Check sheet for the modelled part. Datum: model origin and axes. Units: mm. Face numbers are marked on the shaded views. A direction names the side the tool comes from. Round coordinates to 2 decimals unless told otherwise and drop trailing zeros. Write each loop counter-clockwise with the first axis right and the second up, starting at its lowest first coordinate (ties: lowest second). Pieces come first, ordered by that corner, then holes. Notation, with made-up numbers: (84, 12.5) -> (141, 12.5) arc R29 cw to (141, 36.5) -> close; hole circle Ø9 at (-19.75, 87). An arc over 180 degrees is marked (long way). Write item = value, one per line.
from build123d import *

# Parameters (mm, degrees)
F0_W           = 21
F0_H           = 36.8
F0_R           = 2
F1_DEPTH       = 0.8
F0_W_2         = 5
F2_DEPTH       = 13.5
F5_R           = 6.35
F6_D           = 5
F6_CBORE_D     = 9.5
F6_CBORE_DEPTH = 4.2
F7_W           = 10.5
F7_H           = 2
F7_R           = 2
F8_DEPTH       = 2
F9_DEPTH       = 6.35
F10_T4_DEPTH   = 35.8364431643
F10_T9_DEPTH   = 35.8364431643
F11_W          = 6.8
F11_H          = 6.8
F12_DEPTH      = 2
F13_R          = 0.99999


# Not quite as in the source:
# - a fillet or chamfer that OpenCascade refuses, or shapes differently, is made with other operations: its cross-section is extruded or revolved along the edge and cut away or added
# - a fillet or chamfer is up to 0.001 mm smaller than in the source, because OpenCascade refuses the exact size


with BuildPart() as f1:
    # F0 (on Top) → F1 (new body)
    with BuildSketch(Plane.XY):
        Rectangle(F0_W, F0_H)
        with Locations((-6.35, -12.7)):
            Circle(F0_R, mode=Mode.SUBTRACT)
        with Locations((6.35, -12.7)):
            Circle(F0_R, mode=Mode.SUBTRACT)
        with Locations((-6.35, 12.7)):
            Circle(F0_R, mode=Mode.SUBTRACT)
        with Locations((6.35, 12.7)):
            Circle(F0_R, mode=Mode.SUBTRACT)
    extrude(amount=F1_DEPTH)

    # F0 (on Top) → F2 (join)
    with BuildSketch(Plane.XY):
        with Locations((-13, 0)):
            Rectangle(F0_W_2, F0_H)
    extrude(amount=F2_DEPTH)

    # F5
    f5_edges = [f1.edges().sort_by_distance(p)[0] for p in [
        (-13, -18.4, 13.5),
        (-13, 18.4, 13.5),
    ]]
    fillet(f5_edges, radius=F5_R)

    # F6 (through all)
    with Locations(Plane.YZ.offset(-10.5)):
        with Locations((0, 7.15)):
            CounterBoreHole(F6_D / 2, F6_CBORE_D / 2, F6_CBORE_DEPTH)

    # F7 (on face) → F8 (join)
    with BuildSketch(Plane.XY.offset(0.8)):
        with Locations((-5.25, -17.4)):
            Rectangle(F7_W, F7_H)
        Polygon((-10.5, -16.4), (0, -16.4), (0, -18.4), (10.5, -18.4), (10.5, -7), (-10.5, -7), align=None)
        Polygon((-10.5, 16.4), (-10.5, 7), (10.5, 7), (10.5, 18.4), (0, 18.4), (0, 16.4), align=None)
        with Locations((-6.35, 12.7)):
            Circle(F7_R, mode=Mode.SUBTRACT)
        with Locations((6.35, 12.7)):
            Circle(F7_R, mode=Mode.SUBTRACT)
    extrude(amount=F8_DEPTH)

    # F7 (on face) → F9 (join)
    with BuildSketch(Plane.XY.offset(0.8)):
        with Locations((-5.25, -17.4)):
            Rectangle(F7_W, F7_H)
        with Locations((-5.25, 17.4)):
            Rectangle(F7_W, F7_H)
    extrude(amount=F9_DEPTH)

    # F10: chamfer of 6.35 x 6.5756174926 on 2 edges, made by hand


with BuildPart() as f10_tool2:
    # F10_s3 → F10_t4 (new body)
    with BuildSketch(Plane.XZ.offset(35.3182215821)):
        Polygon((-6.5756174926, 7.15), (0, 0.8), (0, 7.15), align=None)
    extrude(amount=-F10_T4_DEPTH)

    split(bisect_by=Plane.XY.offset(2.8), keep=Keep.TOP)


with BuildPart() as f1_1:
    add(f1.part)

    # F10_t1: cut F10_tool2
    add(f10_tool2.part, mode=Mode.SUBTRACT)


with BuildPart() as f10_tool7:
    # F10_s8 → F10_t9 (new body)
    with BuildSketch(Plane.XZ.offset(0.5182215821)):
        Polygon((-6.35, 7.15), (0, 0.5743825074), (0, 7.15), align=None)
    extrude(amount=-F10_T9_DEPTH)

    split(bisect_by=Plane.XY.offset(2.8), keep=Keep.TOP)


with BuildPart() as f1_2:
    add(f1_1.part)

    # F10_t6: cut F10_tool7
    add(f10_tool7.part, mode=Mode.SUBTRACT)

    # F11 (on face) → F12 (cut)
    with BuildSketch(Plane.XY.offset(2.8)):
        with Locations((-6.35, -12.7)):
            Rectangle(F11_W, F11_H)
        with Locations((6.35, -12.7)):
            Rectangle(F11_W, F11_H)
        with Locations((-6.35, 12.7)):
            Rectangle(F11_W, F11_H)
        with Locations((6.35, 12.7)):
            Rectangle(F11_W, F11_H)
    extrude(amount=-F12_DEPTH, mode=Mode.SUBTRACT)

    # F13 (radius 1 in the source; OpenCascade refuses exactly that, so slightly less here)
    f13_edges = [f1_2.edges().sort_by_distance(p)[0] for p in [
        (10.5, -18.4, 1.4),
        (10.5, 18.4, 1.4),
        (-15.5, -18.4, 3.575),
        (0, 7, 0.8),
        (0, -7, 0.8),
        (0, 7, 2.8),
        (0, -7, 2.8),
        (-15.5, 0, 13.5),
        (-15.5, -16.540128, 11.640128),
        (-15.5, 16.540128, 11.640128),
        (-15.5, 18.4, 3.575),
    ]]
    fillet(f13_edges, radius=F13_R)


solid = f1_2.part
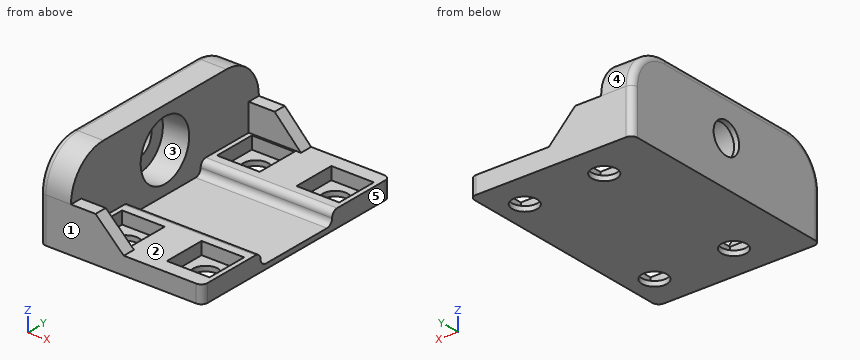
(1) Sectioned sample at D-D on x = -11.25. Enter the section's corners in (y, z), then the cut area to 3 significant figures.
Worked answers:
outline = (-18.4, 0) -> (18.4, 0) -> (18.4, 7.15) arc R6.35 ccw to (12.05, 13.5) -> (-12.05, 13.5) arc R6.35 ccw to (-18.4, 7.15) -> close; hole circle Ø9.5 at (0, 7.15)
area = 409 mm²
(2) Sectioned sample at B-B on x = 6.35. Count the separate pieces of the cut face and the enclosed holes in it, then the cut area to 3 significant figures.
Worked answers:
separate_pieces = 3
enclosed_holes = 0
area = 41.4 mm²
(3) Access from +Z, -Z, +X, -X, +Y, -Y to the whole of each face (thin tool, end or side, straight path). Record for the marked faces 1 and 2.
Worked answers:
face_1 = +Z, -Z, +X, -X, -Y
face_2 = +Z, +X
(4) Sectioned sample at C-C on y = -11.5. Enter the section's corners in (x, z).
Worked answers:
outline = (-15.5, 0) -> (-7.95, 0) -> (-7.95, 0.8) -> (-9.75, 0.8) -> (-9.75, 2.8) -> (-10.5, 2.8) -> (-10.5, 13.5) -> (-14.5, 13.5) arc R1 ccw to (-15.5, 12.5) -> close; (-4.75, 0) -> (4.75, 0) -> (4.75, 0.8) -> (2.95, 0.8) -> (2.95, 2.8) -> (-2.95, 2.8) -> (-2.95, 0.8) -> (-4.75, 0.8) -> close; (7.95, 0) -> (10.5, 0) -> (10.5, 2.8) -> (9.75, 2.8) -> (9.75, 0.8) -> (7.95, 0.8) -> close
(5) Sectioned sample at A-A on y = 0. Enter the section's corners in (x, z).
Worked answers:
outline = (-15.5, 0) -> (10.5, 0) -> (10.5, 0.8) -> (-10.5, 0.8) -> (-10.5, 2.4) -> (-14.7, 2.4) -> (-14.7, 4.65) -> (-15.5, 4.65) -> close; (-15.5, 9.65) -> (-14.7, 9.65) -> (-14.7, 11.9) -> (-10.5, 11.9) -> (-10.5, 13.5) -> (-14.5, 13.5) arc R1 ccw to (-15.5, 12.5) -> close
(6) Go/stop test with flat-tipped pins: P1, Ø4.5, axis at x = 6.35, y = -12.7, coming from the -Z side; P2, Ø6.5, axis at x = -6.35, y = 12.7, coming from the +Z side; P3, Ø8, axis at x = -2, y = -6, coming from the +Z side; P4, Ø1, axis at x = -12, z = 11, coming from the -Y side. Record where each tip stops, or that it passes through.
Worked answers:
P1 = 0
P2 = 0.8
P3 = 2.8
P4 = -17.44
(7) Material ranges on L1, parallel to X at y = 12.7, z = 0.65; L2, parallel to Y at x = -6.35, z = 0.4; L3, parallel to Y at x = 7.5, z = 1.5, recorded low to high. Write a range as [from, to].
Worked answers:
L1 = [-15.5, -8.35], [-4.35, 4.35], [8.35, 10.5]
L2 = [-18.4, -14.7], [-10.7, 10.7], [14.7, 18.4]
L3 = [-18.4, -16.1], [-9.3, -6.95], [6.95, 9.3], [16.1, 18.4]
(8) Release check for a two-part mould opening along Y. For the marked faces 3, 4 and 5 record: pulls with the +Y half, pulls with the -Y half, needs draft (parallel to the pull), parting line crosses it, or undercut.
Worked answers:
face_3 = undercut
face_4 = pulls with the +Y half
face_5 = needs draft
